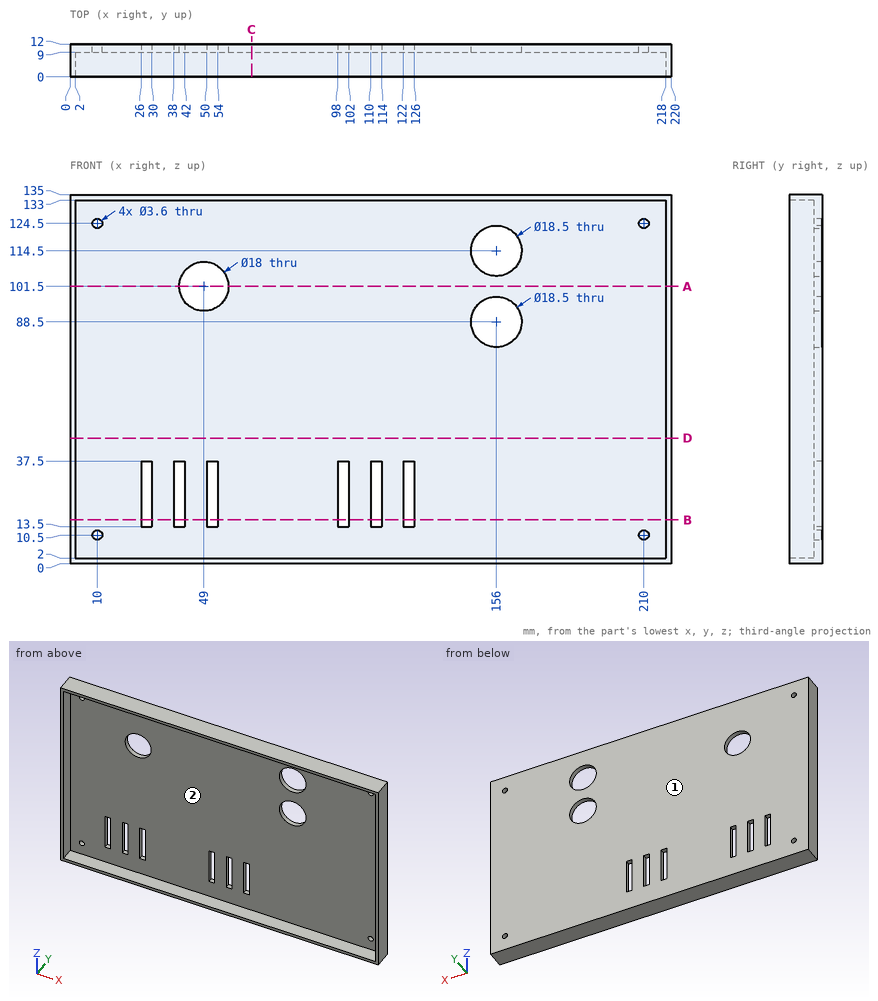
Design review of the part shown in the three views and the two pictorial views. Dimensions are in mm from the part's minimum x, y and z. Round coordinates to 2 decimals unless told otherwise and drop trailing zeros. Order: outer loops, then holes, each group sorted by start corner. A loop starts at its lowest first (then second) coordinate and runs counter-clockwise, first axis right, second up.
Item 1: Draft analysis for pull direction Z (two halves, no side actions). For the marked faces 1 and 2, state which applies: released by +Z, released by -Z, zero draft, split by the parting line, or undercut.
Working result:
face 1: zero draft
face 2: undercut
Item 2: Add section D-D, the plane z = 46. State the section outline as (x, y) points, and give its area (3 significant figures).
Working result:
outline: (0, 0) - (2, 0) - (2, 9) - (218, 9) - (218, 0) - (220, 0) - (220, 12) - (0, 12) - close
area: 696 mm2
Item 3: To check wall thickness, follow probe 1 along Z at (x, y) = (156, 9.9); probe 2 along Z at (x, y) = (210, 10.7); probe 3 along X at (y, z) = (9.9, 10.5). State the ranges of each line that lie inside material, in increasing order.
Working result:
probe 1: z = 0 to 79.25, 97.75 to 105.25, 123.75 to 135
probe 2: z = 0 to 8.7, 12.3 to 122.7, 126.3 to 135
probe 3: x = 0 to 8.2, 11.8 to 208.2, 211.8 to 220
Item 4: Add section A-A, the plane z = 101.5. State the section outline as (x, y) points.
Working result:
outline: (0, 0) - (2, 0) - (2, 9) - (40, 9) - (40, 12) - (0, 12) - close; (58, 9) - (218, 9) - (218, 0) - (220, 0) - (220, 12) - (58, 12) - close
Item 5: For pin 1 (16.5 mm diameter, centred on x = 156, z = 114.5, fed in from +Y), flat-tipped, find the tip position at first contact; note if it passes through.
Working result:
pin 1: passes through
Item 6: Add section C-C, the plane x = 66.5. State the section outline as (y, z) points.
Working result:
outline: (0, 0) - (12, 0) - (12, 135) - (0, 135) - (0, 133) - (9, 133) - (9, 2) - (0, 2) - close
Item 7: Add section B-B, the plane z = 16. Count the separate pieces of the cut face and the enclosed holes in it, and give its area (3 significant figures).
Working result:
separate pieces: 7
enclosed holes: 0
area: 624 mm2
